Work out the finished part from the listing and answer in its coordinate system (mm). A direction names the side the tool comes from. Round coordinates to 2 decimals unless told otherwise and drop trailing zeros. Write each loop counter-clockwise with the first axis right and the second up, starting at its lowest first coordinate (ties: lowest second). Pieces come first, ordered by that corner, then holes. Notation, with made-up numbers: (14.25, 87) -> (68.25, 87) arc R7 ccw to (68.25, 91) -> close; hole circle Ø7 at (-21, -20.5). An arc over 180 degrees is marked (long way). Answer as a JSON object with one key per item and string values. Group by question number.
from build123d import *

# Parameters (mm, degrees)
SKETCH001_R  = 7.773503
POCKET_DEPTH = 29.001
CHAMFER_SIZE = 1


with BuildPart() as part:
    # Sketch → Revolution (revolve)
    with BuildSketch(Plane.XZ):
        Polygon((0, 4), (5, 4), (6, 3.533692), (6, 0.15), (4.44, 0.15), (4.44, 0), (3, 0), (3, -25), (0, -25), align=None)
    revolve(axis=Axis((0, 0, 0), (0, 0, 1)))

    # Sketch001 → Pocket (cut, through all)
    with BuildSketch(Plane(origin=(0, 0, 4), x_dir=(-1, 0, 0), z_dir=(0, 0, 1))):
        Circle(SKETCH001_R)
        Polygon((-2.886751, 5), (2.886751, 5), (5.773503, 0), (2.886751, -5), (-2.886751, -5), (-5.773503, 0), align=None, mode=Mode.SUBTRACT)
    extrude(amount=-POCKET_DEPTH, mode=Mode.SUBTRACT)

    # Chamfer
    chamfer_edges = [part.edges().sort_by_distance(p)[0] for p in [
        (-3, 0, -25),
    ]]
    chamfer(chamfer_edges, length=CHAMFER_SIZE)


solid = part.part
1) A tool of negligible diameter and unlimited length cuts with its end or side. For faces 1 (the face through (0, 0, 4)), 2 (the face through (1, -3, 0)), from which of +Z, -Z, +X, -X, +Y, -Y can it reach the whole face along a straight path? Write none if from no direction.
2) A cutting plane is placed at A-A on z = 2. Determine the outline of the cut face in (x, y), plus the area to 3 significant figures.
3) A cutting plane is placed at B-B on z = -22. Determine the outline of the cut face in (x, y), plus the area to 3 significant figures.
4) Each of these flat-tipped pins is pushed along its axis until it touches: P1, Ø6, axis at x = -2.5, z = -6.5, coming from the +Y side; P2, Ø2, axis at y = 2.5, z = -10.5, coming from the +X side; P3, Ø1, axis at y = -2.5, z = -17, coming from the +X side. Where does it stop, or does it pass through?
5) Straight lines are drawn through the part: L1, parallel to Z at x = -4, y = -0.5; L2, parallel to X at y = 0.5, z = -21; L3, parallel to Z at x = 1.75, y = 1.5. For each, find the intervals that lie inside material, in ascending order.
Established:
{
 "1": {"face 1": "+Z, +X, -X, +Y, -Y", "face 2": "-Z"},
 "2": {"outline": "(-5.77, 0) -> (-2.89, -5) -> (2.89, -5) -> (5.77, 0) -> (2.89, 5) -> (-2.89, 5) -> close", "area": "86.6 mm²"},
 "3": {"outline": "circle Ø6 at (0, 0)", "area": "28.3 mm²"},
 "4": {"P1": "stops at y = 3", "P2": "stops at x = 2.6", "P3": "stops at x = 2.24"},
 "5": {"L1": "z = 0 to 4", "L2": "x = -2.96 to 2.96", "L3": "z = -24.7 to 4"}
}
